Autodesk Fusion 360 part; units mm, degrees
sketch "Sketch1" plane through (0, 0, 0) normal (0, 0, 1) x (1, 0, 0)
  circle A0 centre (26, 26) radius 1.5
  circle A1 centre (6, 6) radius 1.5
  circle A2 centre (6, 26) radius 1.5
  line L0 (0, 0) -> (32, 0)
  circle A3 centre (26, 6) radius 1.5
  line L1 (32, 32) -> (0, 32)
  line L2 (0, 32) -> (0, 0)
  line L3 (32, 0) -> (32, 32)
  dimension "d5" = 20
  dimension "d6" = -20
  dimension "d7" = 32
  dimension "d8" = 32
  dimension "d9" = 3
  dimension "d10" = 6
  dimension "d11" = 6
extrude "Extrude1" add sketch "Sketch1" along normal blind 14
sketch "Sketch2" plane through (32, 0, 0) normal (1, 0, 0) x (0, 1, 0)
  line L0 (0, 0) -> (32, 0)
  line L1 (32, 0) -> (32, 14)
  line L2 (32, 14) -> (0, 14)
  line L3 (0, 14) -> (0, 0)
  line L4 (16, 14) -> (16, 0) construction
  line L5 (0, 7) -> (32, 7) construction
  circle A0 centre (16, 7) radius 3
  dimension "d14" = 6
extrude "Extrude2" cut sketch "Sketch2" against normal up to surface (32 mm away) contours A0
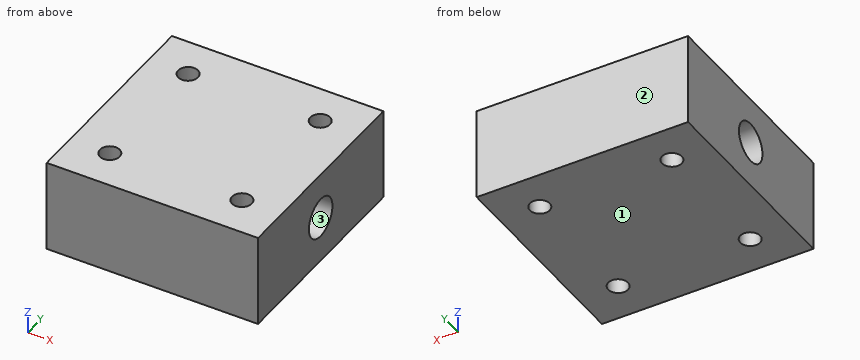
Geometry: final body of the model. Coordinates: model frame, mm. Face numbers are marked on the shaded views. Round coordinates to 2 decimals unless told otherwise and drop trailing zeros. Order: outer loops, then holes, each group sorted by start corner. A loop starts at its lowest first (then second) coordinate and runs counter-clockwise, first axis right, second up.
Q1. Section C-C, the plane y = 6. Output: boundary loops of the cut face in (x, z).
Result sheet:
outline: (0, 0) - (4.5, 0) - (4.5, 14) - (0, 14) - close; (7.5, 0) - (24.5, 0) - (24.5, 14) - (7.5, 14) - close; (27.5, 0) - (32, 0) - (32, 14) - (27.5, 14) - close
Q2. Material intervals for probe 1 along Y at (x, z) = (6, 3); probe 2 along Z at (x, y) = (25, 16); probe 3 along X at (y, z) = (5, 9.25), sorted ascending.
Result sheet:
probe 1: y = 0 to 4.5, 7.5 to 24.5, 27.5 to 32
probe 2: z = 0 to 4, 10 to 14
probe 3: x = 0 to 4.88, 7.12 to 24.88, 27.12 to 32
Q3. Section B-B, the plane y = 16. Output: boundary loops of the cut face in (x, z).
Result sheet:
outline: (0, 0) - (32, 0) - (32, 4) - (0, 4) - close; (0, 10) - (32, 10) - (32, 14) - (0, 14) - close
Q4. Section D-D, the plane z = 10.5. Output: boundary loops of the cut face in (x, y), and give its area (3 significant figures).
Result sheet:
outline: (0, 0) - (32, 0) - (32, 32) - (0, 32) - close; hole circle Ø3 at (6, 6); hole circle Ø3 at (6, 26); hole circle Ø3 at (26, 6); hole circle Ø3 at (26, 26)
area: 996 mm2
Q5. Section A-A, the plane x = 6. Output: boundary loops of the cut face in (y, z), and give its area (3 significant figures).
Result sheet:
outline: (0, 0) - (4.5, 0) - (4.5, 14) - (0, 14) - close; (7.5, 0) - (24.5, 0) - (24.5, 14) - (7.5, 14) - close; (27.5, 0) - (32, 0) - (32, 14) - (27.5, 14) - close; hole circle Ø6 at (16, 7)
area: 336 mm2
Q6. Mould query, pull axis Z, two halves, no side actions, for the marked faces 1, 2 and 3. Classes: released by +Z, released by -Z, zero draft, split by the parting line, or undercut.
Result sheet:
face 1: released by -Z
face 2: zero draft
face 3: undercut
